Source: three-view drawing plus pictorial views. Frame: mm from the lowest corner of the part. Give positions to 0.01 mm unless a question says otherwise; leave off trailing zeros. Order: outer loops, then holes, each group sorted by start corner. A loop starts at its lowest first (then second) coordinate and runs counter-clockwise, first axis right, second up.
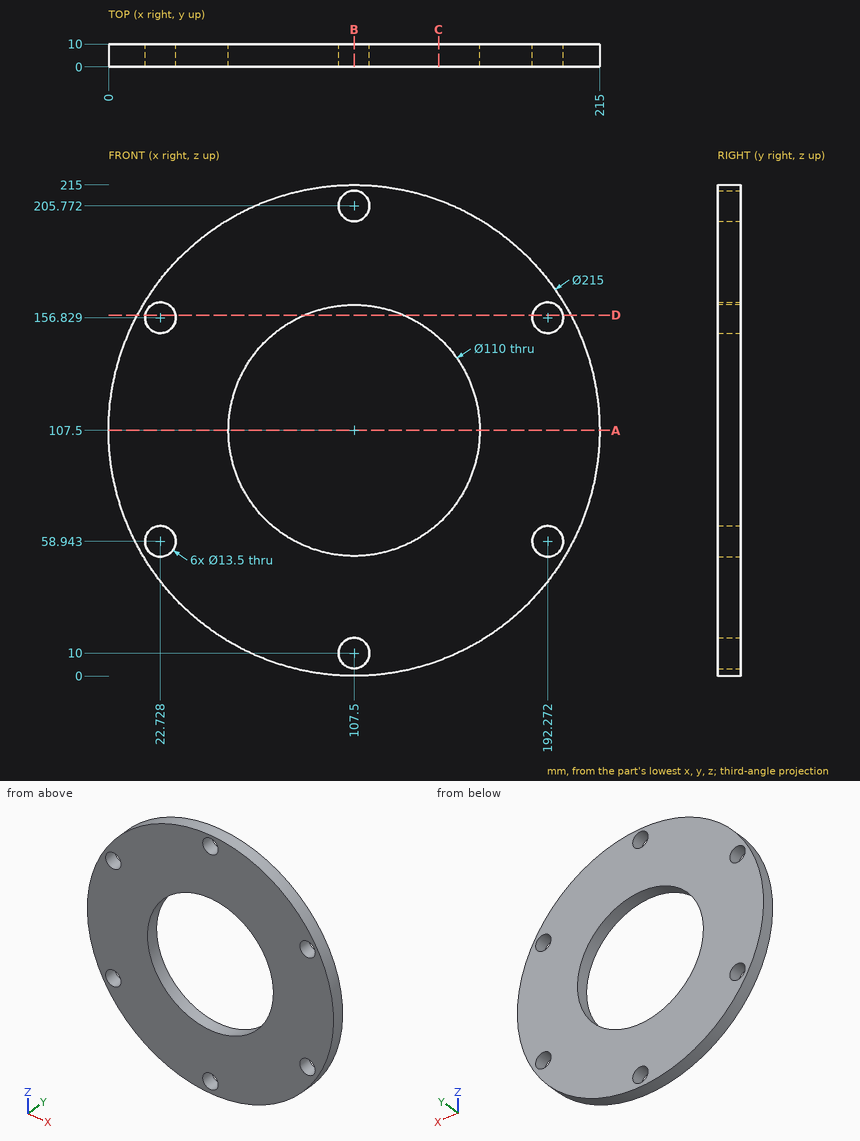
1) Section query A-A on z = 107.5. Output: boundary loops of the cut face in (x, y).
Checks:
outline: (0, 0) - (52.5, 0) - (52.5, 10) - (0, 10) - close; (162.5, 0) - (215, 0) - (215, 10) - (162.5, 10) - close
2) Section query B-B on x = 107.5. Output: boundary loops of the cut face in (y, z).
Checks:
outline: (0, 0) - (10, 0) - (10, 3.25) - (0, 3.25) - close; (0, 16.75) - (10, 16.75) - (10, 52.5) - (0, 52.5) - close; (0, 162.5) - (10, 162.5) - (10, 199.02) - (0, 199.02) - close; (0, 212.52) - (10, 212.52) - (10, 215) - (0, 215) - close
3) Section query C-C on x = 144.5. Output: boundary loops of the cut face in (y, z).
Checks:
outline: (0, 6.57) - (10, 6.57) - (10, 66.81) - (0, 66.81) - close; (0, 148.19) - (10, 148.19) - (10, 208.43) - (0, 208.43) - close
4) First-contact query: pin 1 Ø8 at (x, z) = (160.5, 163) entering from -Y; pin 2 Ø3 at (x, y) = (177, 2) entering from -Z; pin 3 Ø8 at (x, z) = (107.5, 10) entering from +Y; pin 4 Ø1 at (y, z) = (7, 27) entering from +X. Flat tips, straight axial feed; report the tip coordinate or a pass-through.
Checks:
pin 1: stops at y = 0
pin 2: stops at z = 24.24
pin 3: passes through
pin 4: stops at x = 179.31
5) Section query D-D on z = 158. Output: boundary loops of the cut face in (x, y), and give its area (3 significant figures).
Checks:
outline: (12.6, 0) - (16.08, 0) - (16.08, 10) - (12.6, 10) - close; (29.38, 0) - (85.71, 0) - (85.71, 10) - (29.38, 10) - close; (129.29, 0) - (185.62, 0) - (185.62, 10) - (129.29, 10) - close; (198.92, 0) - (202.4, 0) - (202.4, 10) - (198.92, 10) - close
area: 1,200 mm2
6) Ray query, L1, parallel to Z at x = 111.5, y = 7.75 (1 decimal); L2, parallel to X at y = 2.25, z = 108.5 (1 decimal); L3, parallel to Z at x = 27, y = 7 (1 decimal). Return the intervals inside material, ascending.
Checks:
L1: z = 0.1 to 4.6, 15.4 to 52.6, 162.4 to 200.3, 211.2 to 214.9
L2: x = 0 to 52.5, 162.5 to 215
L3: z = 36.3 to 53.7, 64.2 to 151.6, 162.1 to 178.7
